Check sheet for the drawn part. Datum: minimum x, y, z corner. Units: mm. A direction names the side the tool comes from. Coordinates: 2 decimals unless noted, no trailing zeros. Order: outer loops, then holes, each group sorted by start corner. A loop starts at its lowest first (then second) coordinate and runs counter-clockwise, first axis right, second up. Notation, with made-up numbers: (-23, 53.25) - (27, 53.25) arc R30 ccw to (27, 75.25) - close; hole circle Ø1 at (-15, 62.5). An arc over 180 degrees is marked (long way). Return JSON: item names as keys, results as strings. Group by question number.
Item 1: Section check A-A on x = 7. Give the number of separate pieces and of enclosed holes in the cut face, then the cut area to 3 significant figures.
Item 2: Section check B-B on y = 28.85. Enter the section's corners in (x, z).
Item 3: Scan lines: probe 1 along Y at (x, z) = (7, 4.05); probe 2 along Y at (x, z) = (1, 17.5); probe 3 along Z at (x, y) = (11, 40) (1 decimal). Record each from-to range of solid material in increasing order.
Item 4: Draft check along Y on the marked faces 4, 5, 6 and 7. Enter one of: pulls with the +Y half, pulls with the -Y half, needs draft (parallel to the pull), parting line crosses it, or undercut.
Item 5: Section check C-C on z = 12.5. Enter the section's corners in (x, y), then the cut area to 3 significant figures.
Item 6: Gauge pin test, flat ends, axial feed: pin 1 (2.5 mm diameter, centred on x = 7, y = 11.35, fed in from -Z); pin 2 (0.8 mm diameter, centred on x = 6, z = 0.5, fed in from +Y); pin 3 (2 mm diameter, centred on x = 2.5, y = 39.5, fed in from +Z) (1 decimal). Record the tip position at first contact, or that the pin passes through.
Item 7: Tool access check on the marked faces 1, 2 and 3. Record the directions out of +Z, -Z, +X, -X, +Y, -Y that give a thin tool (end or side, any length) a straight path to the whole face; none if there is none.
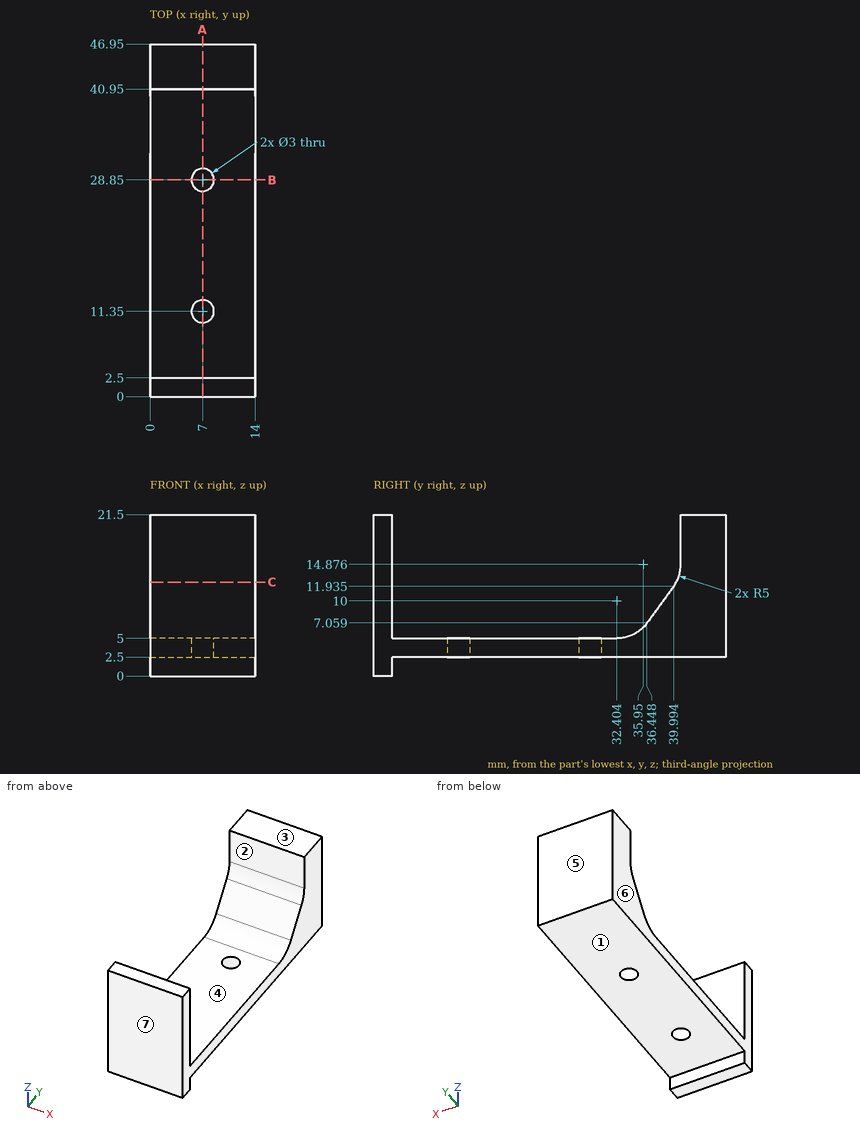
Computed:
{
 "1": {"separate pieces": "3", "enclosed holes": "0", "area": "275 mm²"},
 "2": {"outline": "(0, 2.5) - (5.5, 2.5) - (5.5, 5) - (0, 5) - close; (8.5, 2.5) - (14, 2.5) - (14, 5) - (8.5, 5) - close"},
 "3": {"probe 1": "y = 0 to 9.85, 12.85 to 27.35, 30.35 to 46.95", "probe 2": "y = 0 to 2.5, 40.95 to 46.95", "probe 3": "z = 2.5 to 11.9"},
 "4": {"face 4": "undercut", "face 5": "pulls with the +Y half", "face 6": "needs draft", "face 7": "pulls with the -Y half"},
 "5": {"outline": "(0, 0) - (14, 0) - (14, 2.5) - (0, 2.5) - close; (0, 40.35) - (14, 40.35) - (14, 46.95) - (0, 46.95) - close", "area": "127 mm²"},
 "6": {"pin 1": "passes through", "pin 2": "stops at y = 2.5", "pin 3": "stops at z = 12.8"},
 "7": {"face 1": "-Z, +X, -X, +Y", "face 2": "+Z, +X, -X", "face 3": "+Z, +X, -X, +Y, -Y"}
}
